Input: dimensioned drawing with shaded views. Units: mm. Origin: part minimum x, y, z. A direction names the side the tool comes from. Coordinates: 2 decimals unless noted, no trailing zeros. Order: outer loops, then holes, each group sorted by start corner. A loop starts at its lowest first (then second) coordinate and runs counter-clockwise, first axis right, second up.
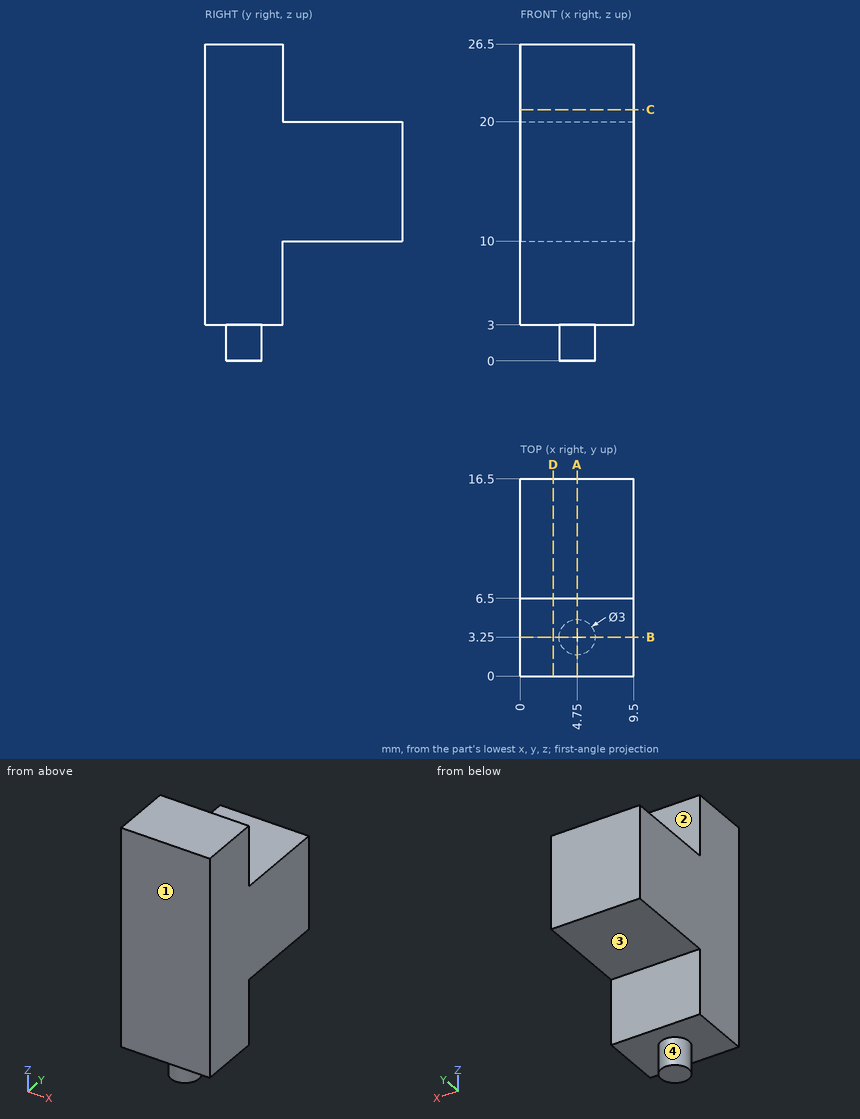
1. Section query A-A on x = 4.75. Return loops of the section in (y, z), plus the area to 3 significant figures.
Findings:
outline: (0, 3) - (1.75, 3) - (1.75, 0) - (4.75, 0) - (4.75, 3) - (6.5, 3) - (6.5, 10) - (16.5, 10) - (16.5, 20) - (6.5, 20) - (6.5, 26.5) - (0, 26.5) - close
area: 262 mm2
2. Pin query (flat end, axial travel): P1, Ø1, axis at x = 4.5, y = 8.5, coming from the +Z side; P2, Ø5.5, axis at x = 2.5, z = 7, coming from the +Y side. Return the tip coordinate at first contact, or that it passes through.
Findings:
P1: stops at z = 20
P2: stops at y = 6.5
3. Access query for the marked faces 1, 2, 3 and 4. Directions: +Z, -Z, +X, -X, +Y, -Y. A direction counts if a zero-diameter tool reaches every point of the face in a straight line with its end or side. Return the directions, or none.
Findings:
face 1: +Z, -Z, +X, -X, -Y
face 2: +Z, +X, -X, +Y
face 3: -Z, +X, -X, +Y
face 4: -Z
4. Section query C-C on z = 21. Return loops of the section in (x, y), plus the area to 4 significant figures.
Findings:
outline: (0, 0) - (9.5, 0) - (9.5, 6.5) - (0, 6.5) - close
area: 61.75 mm2
5. Ray query, line 1 (Y direction, x = 3, z = 22.5); line 2 (Z direction, x = 4, y = 7); line 3 (Z direction, x = 7.5, y = 1.5). Return the intervals inside material, ascending.
Findings:
line 1: y = 0 to 6.5
line 2: z = 10 to 20
line 3: z = 3 to 26.5
6. Section query D-D on x = 2.75. Return loops of the section in (y, z).
Findings:
outline: (0, 3) - (6.5, 3) - (6.5, 10) - (16.5, 10) - (16.5, 20) - (6.5, 20) - (6.5, 26.5) - (0, 26.5) - close
7. Section query B-B on y = 3.25. Return loops of the section in (x, z), plus the area to 3 significant figures.
Findings:
outline: (0, 3) - (3.25, 3) - (3.25, 0) - (6.25, 0) - (6.25, 3) - (9.5, 3) - (9.5, 26.5) - (0, 26.5) - close
area: 232 mm2
